Check sheet for the modelled part. Datum: model origin and axes. Units: mm. Give positions to 0.01 mm unless a question says otherwise; leave off trailing zeros. Order: outer loops, then holes, each group sorted by start corner. A loop starts at its lowest first (then second) coordinate and runs counter-clockwise, first axis right, second up. Notation, with made-up numbers: (-39, -36) -> (15, -36) arc R26 cw to (15, -2) -> close; hole circle Ø2 at (12, 7). An arc over 180 degrees is marked (long way). One line per question, with ' | ' between items.
Autodesk Inventor part; units mm, degrees
ref_plane "YZ Plane" through (0, 0, 0) normal (1, 0, 0) x (0, 1, 0)
ref_plane "XZ Plane" through (0, 0, 0) normal (0, 1, 0) x (-1, 0, 0)
ref_plane "XY Plane" through (0, 0, 0) normal (0, 0, 1) x (1, 0, 0)
sketch "Sketch2" plane through (0, 0, 0) normal (0, 0, 1) x (1, 0, 0)
  line L0 (-256.5, 106.2458) -> (-106.2458, 256.5)
  line L1 (-106.2458, 256.5) -> (106.2458, 256.5)
  line L2 (106.2458, 256.5) -> (256.5, 106.2458)
  line L3 (256.5, 106.2458) -> (256.5, -106.2458)
  line L4 (256.5, -106.2458) -> (106.2458, -256.5)
  line L5 (106.2458, -256.5) -> (-106.2458, -256.5)
  line L6 (-106.2458, -256.5) -> (-256.5, -106.2458)
  line L7 (-256.5, -106.2458) -> (-256.5, 106.2458)
  circle A0 centre (0, 0) radius 194.5
  point P0 (0, 256.5)
  dimension "d23" = 513
  dimension "d26" = 389
extrude "Plate1" add sketch "Sketch2" against normal blind 3
sketch "Sketch4" plane through (0, 0, 0) normal (0, 0, 1) x (1, 0, 0)
  circle A0 centre (0, 214.5) radius 6.25
  circle A1 centre (0, 0) radius 194.5
  dimension "d16" = 12.5
  dimension "d17" = 214.5
extrude "Extrusion1" cut sketch "Sketch4" against normal up to surface (3 mm away) contours A0
pattern_circular "Circular Pattern1" count 8 over 360 about axis through (0, 0, -10) along (0, 0, 1) of "Extrusion1"
equation "\"d23\" = Барабан_габарит_по_кассетам"
equation "\"d26\" = Вал_ось_диаметр_КОРМА"
equation "\"d15\" = Thickness"
equation "\"BendRadius\" = Thickness"
equation "\"BendReliefWidth\" = Thickness"
equation "\"BendReliefDepth\" = 0.5 * Thickness"
equation "\"CornerReliefSize\" = 4 * Thickness"
equation "\"MinimumRemnant\" = 2 * Thickness"
equation "\"TransitionRadius\" = BendRadius"
equation "\"JacobiRadiusSize\" = BendRadius"
equation "\"GapSize\" = Thickness"
properties part number "ДМФ 01 22 Барабан торец КОРМА v2.0"
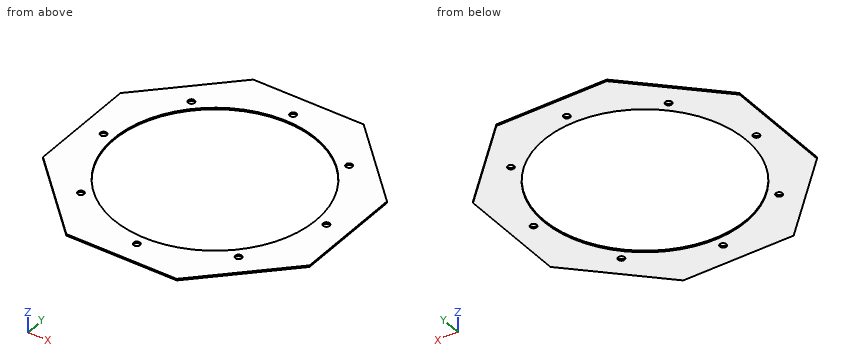
Q1. Section check A-A (y = 0). Enter the section's corners in (x, z), and give its area (3 significant figures).
Result sheet:
outline: (-256.5, -3) -> (-220.75, -3) -> (-220.75, 0) -> (-256.5, 0) -> close; (-208.25, -3) -> (-194.5, -3) -> (-194.5, 0) -> (-208.25, 0) -> close; (194.5, -3) -> (208.25, -3) -> (208.25, 0) -> (194.5, 0) -> close; (220.75, -3) -> (256.5, -3) -> (256.5, 0) -> (220.75, 0) -> close | area: 297 mm2
Q2. Thickness scan on line 1 (Y direction, x = 0, z = -1.5); line 2 (Y direction, x = -150, z = -1.2); line 3 (X direction, y = -146, z = -2.7). Record the ranges inside material, lowest first.
Result sheet:
line 1: y = -256.5 to -220.75, -208.25 to -194.5, 194.5 to 208.25, 220.75 to 256.5 | line 2: y = -212.75 to -157.7, -145.65 to -123.82, 123.82 to 145.65, 157.7 to 212.75 | line 3: x = -216.75 to -154.29, -149.05 to -128.51, 128.51 to 149.05, 154.29 to 216.75
Q3. Depth check by flat-ended pin: pin 1 Ø1.5 at (y, z) = (-134.5, -2.5) entering from -X; pin 2 Ø1 at (x, z) = (-142, -2.5) entering from +Y. Enter the tip coordinate at first touch or a pass-through.
Result sheet:
pin 1: stops at x = -229 | pin 2: stops at y = 221.25
Q4. Section check D-D (y = 214.5). Enter the section's corners in (x, z), and give its area (3 significant figures).
Result sheet:
outline: (-148.25, -3) -> (-6.25, -3) -> (-6.25, 0) -> (-148.25, 0) -> close; (6.25, -3) -> (148.25, -3) -> (148.25, 0) -> (6.25, 0) -> close | area: 852 mm2
Q5. Section check C-C (z = -1.3). Count the separate pieces of the cut face and the enclosed holes in it, and give its area (3 significant figures).
Result sheet:
separate pieces: 1 | enclosed holes: 9 | area: 98,200 mm2
